```python
from build123d import *

# Parameters (mm, degrees)
SKETCH1_R           = 10.75
BOSS_EXTRUDE5_DEPTH = 2
SKETCH4_R           = 5
BOSS_EXTRUDE6_DEPTH = 8
CUT_EXTRUDE2_DEPTH  = 0.5
FILLET1_R           = 0.5


with BuildPart() as part:
    # Sketch1 → Boss-Extrude5 (new body)
    with BuildSketch(Plane(origin=(0, 0, 0), x_dir=(1, 0, 0), z_dir=(0, 1, 0))):
        with Locations(Location((-5.408676197, -40.3067379, 0), (0, 0, 270))):
            Circle(SKETCH1_R)
    extrude(amount=BOSS_EXTRUDE5_DEPTH)

    # Sketch4 → Boss-Extrude6 (add)
    with BuildSketch(Plane(origin=(0, 2, 0), x_dir=(1, 0, 0), z_dir=(0, 1, 0))):
        with Locations(Location((-5.408676197, -40.3067379, 0), (0, 0, 270))):
            Circle(SKETCH4_R)
    extrude(amount=BOSS_EXTRUDE6_DEPTH)

    # Sketch5 → Cut-Extrude2 (cut)
    with BuildSketch(Plane.XZ):
        with BuildLine():
            Line((-1.119213117, 44.837068706), (-1.119213117, 43.683222552))
            Line((-1.119213117, 43.683222552), (-5.343972733, 43.683222552))
            Line((-5.343972733, 43.683222552), (-6.023059271, 41.293398834))
            add(Edge.make_bspline(
                [(-6.023059271, 41.293398834), (-5.932156571, 41.326006682), (-5.748327994, 41.391948115), (-5.457355976, 41.457073381), (-5.152680183, 41.494921804), (-4.944776832, 41.500766404), (-4.83916504, 41.503735373)],
                knots=[0, 0, 0, 0, 0.957717051, 1.936749544, 2.951899637, 4, 4, 4, 4], degree=3))
            add(Edge.make_bspline(
                [(-4.83916504, 41.503735373), (-4.692794844, 41.501511705), (-4.405302434, 41.497144096), (-3.984914685, 41.449022779), (-3.584114393, 41.376035058), (-3.203409576, 41.272428706), (-2.84410494, 41.134960143), (-2.503422249, 40.970833678), (-2.183430631, 40.775504615), (-1.886735045, 40.552203964), (-1.617614167, 40.307560211), (-1.380562504, 40.046212071), (-1.18207178, 39.768708327), (-1.016586663, 39.477477761), (-0.89101931, 39.170105093), (-0.800035696, 38.848376848), (-0.744603566, 38.51220008), (-0.73796564, 38.282791456), (-0.734597733, 38.166395629)],
                knots=[0, 0, 0, 0, 1.189422793, 2.336199813, 3.434961192, 4.499048693, 5.538481089, 6.55816476, 7.569214574, 8.581065566, 9.572455183, 10.521863525, 11.44380993, 12.340676557, 13.23887286, 14.135887326, 15.054198869, 16, 16, 16, 16], degree=3))
            add(Edge.make_bspline(
                [(-0.734597733, 38.166395629), (-0.736640177, 38.085517838), (-0.740703434, 37.924618805), (-0.769785303, 37.68553966), (-0.815472566, 37.451064567), (-0.880132404, 37.220499767), (-0.964125821, 36.994808543), (-1.06783674, 36.773146693), (-1.187054465, 36.554434869), (-1.327713423, 36.342988535), (-1.484068604, 36.139863296), (-1.651274877, 35.943889885), (-1.836982388, 35.763848397), (-2.036297248, 35.595294519), (-2.247651639, 35.436933598), (-2.474538943, 35.29216457), (-2.713969847, 35.157576429), (-2.969100544, 35.038319676), (-3.234502949, 34.930569363), (-3.510180209, 34.835095329), (-3.796371201, 34.758164461), (-4.092034227, 34.694367722), (-4.396528465, 34.641310625), (-4.710907901, 34.605736687), (-5.035226874, 34.586116093), (-5.254470616, 34.582498734), (-5.366007989, 34.58065845)],
                knots=[0, 0, 0, 0, 0.892114965, 1.774781853, 2.653165494, 3.525411504, 4.413472142, 5.306650977, 6.223218553, 7.158975213, 8.104883377, 9.050131562, 9.99821726, 10.954651527, 11.928515787, 12.909348305, 13.921788707, 14.956496026, 16.013925213, 17.080882478, 18.172775305, 19.281020983, 20.417001569, 21.581128518, 22.769430922, 24, 24, 24, 24], degree=3))
            add(Edge.make_bspline(
                [(-5.366007989, 34.58065845), (-5.494284486, 34.583063858), (-5.745955956, 34.587783137), (-6.116184202, 34.622034821), (-6.47081652, 34.680178398), (-6.811266316, 34.759884514), (-7.136893236, 34.864233845), (-7.447568471, 34.992564198), (-7.743090523, 35.14314329), (-8.021755023, 35.315119606), (-8.280263283, 35.507749531), (-8.511328327, 35.723822234), (-8.717302907, 35.956398551), (-8.894124812, 36.208989698), (-9.04611222, 36.478757404), (-9.167730863, 36.768695414), (-9.263331665, 37.077407764), (-9.303738659, 37.291837918), (-9.324341322, 37.40117127)],
                knots=[0, 0, 0, 0, 1.156081109, 2.268167895, 3.347613226, 4.39280983, 5.416773159, 6.426003973, 7.419190543, 8.402904802, 9.374262051, 10.319617, 11.249247452, 12.16926304, 13.093442327, 14.034631047, 14.997900376, 16, 16, 16, 16], degree=3))
            Line((-9.324341322, 37.40117127), (-7.695735553, 37.40117127))
            add(Edge.make_bspline(
                [(-7.695735553, 37.40117127), (-7.665938842, 37.29822773), (-7.609424759, 37.102979349), (-7.494386677, 36.837131133), (-7.365578693, 36.610682144), (-7.212981365, 36.424647701), (-7.037244542, 36.271186273), (-6.837886683, 36.140033103), (-6.61753111, 36.018032238), (-6.372231072, 35.91845502), (-6.113028221, 35.8367159), (-5.84405185, 35.778976521), (-5.569406027, 35.74118536), (-5.383493923, 35.736741906), (-5.289886194, 35.734504604)],
                knots=[0, 0, 0, 0, 1.209492624, 2.293990239, 3.264217245, 4.143063212, 4.998087424, 5.889275892, 6.834373525, 7.838714582, 8.874072118, 9.900821757, 10.943052634, 12, 12, 12, 12], degree=3))
            add(Edge.make_bspline(
                [(-5.289886194, 35.734504604), (-5.192324005, 35.737130811), (-5.000016086, 35.74230741), (-4.716910345, 35.773750579), (-4.444965931, 35.830559113), (-4.183508131, 35.908770189), (-3.932477159, 36.008780442), (-3.692754799, 36.132122968), (-3.463766496, 36.276386897), (-3.249014093, 36.441955602), (-3.05146791, 36.623085173), (-2.876018465, 36.816002223), (-2.730880971, 37.023688964), (-2.609082001, 37.239620566), (-2.517761773, 37.468564453), (-2.447455886, 37.705428454), (-2.410200354, 37.954886602), (-2.40427986, 38.124220181), (-2.401264399, 38.210466142)],
                knots=[0, 0, 0, 0, 1.106657597, 2.181367805, 3.225543607, 4.253442955, 5.273050397, 6.28579989, 7.306953151, 8.338528751, 9.35692601, 10.343744444, 11.289304653, 12.224986422, 13.148978842, 14.079003922, 15.021587128, 16, 16, 16, 16], degree=3))
            add(Edge.make_bspline(
                [(-2.401264399, 38.210466142), (-2.40349869, 38.287396604), (-2.407895611, 38.438790134), (-2.444921346, 38.660709645), (-2.50534817, 38.871421278), (-2.586864736, 39.072480407), (-2.697529217, 39.259124567), (-2.828175751, 39.437781279), (-2.985412858, 39.603263585), (-3.164070316, 39.757245811), (-3.36148755, 39.89819609), (-3.579946856, 40.017155777), (-3.812244826, 40.12252931), (-4.062002973, 40.206367726), (-4.32827546, 40.270150154), (-4.610885079, 40.315501078), (-4.910695843, 40.344133926), (-5.116208444, 40.347936099), (-5.22177722, 40.349889219)],
                knots=[0, 0, 0, 0, 0.930198305, 1.830562318, 2.712659836, 3.578217842, 4.446898647, 5.330622017, 6.250663937, 7.201295639, 8.18069732, 9.178676739, 10.205529286, 11.263059576, 12.360199582, 13.514207819, 14.723085422, 16, 16, 16, 16], degree=3))
            add(Edge.make_bspline(
                [(-5.22177722, 40.349889219), (-5.313303916, 40.348222189), (-5.50398839, 40.344749139), (-5.801393829, 40.318860761), (-6.120830833, 40.278998633), (-6.462766686, 40.221835601), (-6.826240906, 40.149976218), (-7.212080245, 40.060704798), (-7.620322897, 39.957040722), (-7.898916934, 39.877831976), (-8.04229004, 39.837068706)],
                knots=[0, 0, 0, 0, 0.763917436, 1.591526851, 2.490253246, 3.450542423, 4.484603654, 5.582488234, 6.755873684, 8, 8, 8, 8], degree=3))
            Line((-8.04229004, 39.837068706), (-6.730190681, 44.837068706))
            Line((-6.730190681, 44.837068706), (-1.119213117, 44.837068706))
        make_face()
    extrude(amount=-CUT_EXTRUDE2_DEPTH, mode=Mode.SUBTRACT)

    # Fillet1
    fillet1_edges = [part.edges().sort_by_distance(p)[0] for p in [
        (-5.408676197, 0, 29.5567379),
        (-5.408676197, 2, 29.5567379),
    ]]
    fillet(fillet1_edges, radius=FILLET1_R)


solid = part.part
```
Can you work these out from the model? Positions are in its coordinate system, mm. Coordinates: 2 decimals unless noted, no trailing zeros. Write each loop counter-clockwise with the first axis right and the second up, starting at its lowest first coordinate (ties: lowest second). Pieces come first, ordered by that corner, then holes. Notation, with made-up numbers: M 20,29 L 32,29 A17 cw 32,38 Z; hole C 4.25,56 d6. An arc over 180 degrees is marked long. Answer as CSV lines item,"result".
Item 1: I'm going to push flat-ended pins straight in: P1, Ø5, axis at x = -10, y = 5, coming from the -Z side; P2, Ø1, axis at x = -9.5, y = 3.5, coming from the +Z side; P3, Ø1.5, axis at x = -7.5, y = 3, coming from the +Z side. Where does each tip first touch, or does it pass through?
Geometry results:
P1,"stops at z = 35.77"
P2,"stops at z = 43.79"
P3,"stops at z = 45.12"
Item 2: Please list where these lines run through material, in increasing order: line 1 along Y through (x, z) = (-9, 44.5); line 2 along X through (y, z) = (1.25, 35); line 3 along Y through (x, z) = (-8, 37.25).
Geometry results:
line 1,"y = 0 to 2"
line 2,"x = -14.76 to 3.94"
line 3,"y = 0.5 to 10"
Item 3: We'd pull the mould along Z, two halves only. Please class faces 1 (the cylindrical face through (-7.324, 5.944, 44.925)), 2 (the flat face through (-3, 2, 45)), 3 (the flat face through (-7.395, 0.246, 42.302)): +Z half, -Z half, draft (parallel to the pull), parting line (faces both ways), or undercut.
Geometry results:
face 1,"parting line"
face 2,"draft"
face 3,"undercut"
Item 4: Imagine slicing it at A-A on y = 3.75. List the corners of the cut face in (x, z) for me.
Geometry results:
outline,"C -5.41,40.31 d10"
